```python
from build123d import *

# Parameters (mm, degrees)
SKETCH1_W                       = 361.95
SKETCH1_H                       = 110.744
BOSS_EXTRUDE1_DEPTH             = 3.175
CUT_EXTRUDE1_DEPTH              = 379.526243028
SKETCH3_W                       = 36.5125
SKETCH3_H                       = 28.575
CUT_EXTRUDE2_DEPTH              = 379.526243028
FILLET1_R                       = 6.35
F_1_4_CLEARANCE_HOLE1_OUTLINE_R = 3.3782
F_1_4_CLEARANCE_HOLE1_DEPTH     = 3.175
CUT_EXTRUDE6_DEPTH              = 3.175


# Read off the part's stored shape, not the designer's step: 1/4 Clearance Hole1, Cut-Extrude6
with BuildPart() as part:
    # Sketch1 → Boss-Extrude1 (new body)
    with BuildSketch(Plane(origin=(0, 0, 0), x_dir=(1, 0, 0), z_dir=(0, 1, 0))):
        with Locations((180.975, 55.372)):
            Rectangle(SKETCH1_W, SKETCH1_H)
    extrude(amount=BOSS_EXTRUDE1_DEPTH)

    # Sketch2 → Cut-Extrude1 (cut, through all)
    with BuildSketch(Plane(origin=(0, 3.175, 0), x_dir=(1, 0, 0), z_dir=(0, 1, 0))):
        Polygon((0, 0), (31.233038214, 110.744), (0, 110.744), align=None)
        Polygon((361.95, 0), (307.33710294, 110.744), (361.95, 110.744), align=None)
    extrude(amount=-CUT_EXTRUDE1_DEPTH, mode=Mode.SUBTRACT)

    # Sketch3 → Cut-Extrude2 (cut, through all)
    with BuildSketch(Plane(origin=(0, 3.175, 0), x_dir=(1, 0, 0), z_dir=(0, 1, 0))):
        with Locations((57.15, 96.4565)):
            Rectangle(SKETCH3_W, SKETCH3_H)
        with Locations((285.75, 96.4565)):
            Rectangle(SKETCH3_W, SKETCH3_H)
    extrude(amount=-CUT_EXTRUDE2_DEPTH, mode=Mode.SUBTRACT)

    # Fillet1
    fillet1_edges = [part.edges().sort_by_distance(p)[0] for p in [
        (75.40625, 1.5875, -82.169),
        (38.89375, 1.5875, -82.169),
        (304.00625, 1.5875, -82.169),
        (267.49375, 1.5875, -82.169),
    ]]
    fillet(fillet1_edges, radius=FILLET1_R)

    # 1/4 Clearance Hole1 outline → 1/4 Clearance Hole1 (cut)
    with BuildSketch(Plane(origin=(0, 0, 0), x_dir=(1, 0, 0), z_dir=(0, 1, 0))):
        with BuildLine():
            ThreePointArc((51.7525, 23.01875), (56.1975, 18.57375), (60.6425, 23.01875))
            Line((60.6425, 23.01875), (60.6425, 27.78125))
            ThreePointArc((60.6425, 27.78125), (56.1975, 32.22625), (51.7525, 27.78125))
            Line((51.7525, 27.78125), (51.7525, 23.01875))
        make_face()
        with Locations((297.65625, 23.314421689)):
            Circle(F_1_4_CLEARANCE_HOLE1_OUTLINE_R)
        with Locations((297.65625, 42.364421689)):
            Circle(F_1_4_CLEARANCE_HOLE1_OUTLINE_R)
        with Locations((45.24375, 23.314421689)):
            Circle(F_1_4_CLEARANCE_HOLE1_OUTLINE_R)
        with Locations((45.24375, 42.364421689)):
            Circle(F_1_4_CLEARANCE_HOLE1_OUTLINE_R)
    extrude(amount=F_1_4_CLEARANCE_HOLE1_DEPTH, mode=Mode.SUBTRACT)

    # Cut-Extrude6 outline → Cut-Extrude6 (cut)
    with BuildSketch(Plane(origin=(0, 0, 0), x_dir=(1, 0, 0), z_dir=(0, 1, 0))):
        with BuildLine():
            ThreePointArc((39.02075, 71.1835), (39.8145, 71.97725), (39.02075, 72.771))
            Line((39.02075, 72.771), (32.41675, 72.771))
            ThreePointArc((32.41675, 72.771), (31.623, 71.97725), (32.41675, 71.1835))
            Line((32.41675, 71.1835), (32.41675, 39.240862815))
            ThreePointArc((32.41675, 39.240862815), (31.623, 38.447112815), (32.41675, 37.653362815))
            Line((32.41675, 37.653362815), (39.02075, 37.653362815))
            ThreePointArc((39.02075, 37.653362815), (39.8145, 38.447112815), (39.02075, 39.240862815))
            Line((39.02075, 39.240862815), (39.02075, 71.1835))
        make_face()
        with BuildLine():
            ThreePointArc((310.48325, 71.1835), (311.277, 71.97725), (310.48325, 72.771))
            Line((310.48325, 72.771), (303.87925, 72.771))
            ThreePointArc((303.87925, 72.771), (303.0855, 71.97725), (303.87925, 71.1835))
            Line((303.87925, 71.1835), (303.87925, 39.240862815))
            ThreePointArc((303.87925, 39.240862815), (303.0855, 38.447112815), (303.87925, 37.653362815))
            Line((303.87925, 37.653362815), (310.48325, 37.653362815))
            ThreePointArc((310.48325, 37.653362815), (311.277, 38.447112815), (310.48325, 39.240862815))
            Line((310.48325, 39.240862815), (310.48325, 71.1835))
        make_face()
    extrude(amount=CUT_EXTRUDE6_DEPTH, mode=Mode.SUBTRACT)


solid = part.part
```
Work out the finished part from the listing and answer in its coordinate system (mm). A direction names the side the tool comes from. Give positions to 0.01 mm unless a question says otherwise; leave off trailing zeros. Order: outer loops, then holes, each group sorted by start corner. A loop starts at its lowest first (then second) coordinate and runs counter-clockwise, first axis right, second up. Notation, with made-up numbers: M 74,-5 L 118,-5 A19 ccw 118,2 Z; hole C 55.5,30.25 d1. An arc over 180 degrees is marked long. Return JSON: item names as keys, results as strings.
1) Each of these flat-tipped pins is pushed along its axis until it touches: pin 1 (1.6 mm diameter, centred on y = 1, z = -26, fed in from +X); pin 2 (1 mm diameter, centred on x = 289, y = 1, fed in from -Z); pin 3 (1 mm diameter, centred on x = 46, z = -41.5, fed in from +Y); pin 4 (1 mm diameter, centred on y = 2, z = -53.5, fed in from +X). Where does it stop, or does it pass through?
Resolved:
{"pin 1": "x = 349.52", "pin 2": "z = -82.17", "pin 3": "through", "pin 4": "x = 335.81"}
2) Section C-C, the plane y = 1.85 is taken. Give the number of separate pieces and of enclosed holes in the cut face, plus the area to 3 significant figures.
Resolved:
{"separate pieces": "1", "enclosed holes": "7", "area": "32,600 mm^2"}
3) Section B-B, the plane z = -61 is taken. Write down the section's boundary in (x, y) (3 decimals).
Resolved:
{"outline": "M 17.204,0 L 32.417,0 L 32.417,3.175 L 17.204,3.175 Z; M 39.021,0 L 303.879,0 L 303.879,3.175 L 39.021,3.175 Z; M 310.483,0 L 331.868,0 L 331.868,3.175 L 310.483,3.175 Z"}
4) A tool of negligible diameter and unlimited length cuts with its end or side. For faces 1 (the flat face through (15.4, 1.6, -54.6)), 2 (the cylindrical face through (73.497, 1.565, -83.98)), from which of +Z, -Z, +X, -X, +Y, -Y can it reach the whole face along a straight path? Write none if from no direction.
Resolved:
{"face 1": "-Z, -X, +Y, -Y", "face 2": "-Z, +Y, -Y"}
5) Straight lines are drawn through the part: line 1 along Z through (x, y) = (298, 2.25); line 2 along X through (y, z) = (0.3, -57); line 3 along X through (y, z) = (1.05, -83). For each, find the intervals that lie inside material, in ascending order. Write a range as [from, to].
Resolved:
{"line 1": "[-82.18, -45.73], [-39, -26.68], [-19.95, 0]", "line 2": "[16.08, 32.42], [39.02, 303.88], [310.48, 333.84]", "line 3": "[23.41, 42.1], [72.2, 270.7], [300.8, 321.02]"}
6) For a pull along X with two mould halves and no side action, classify faces 3 (the flat face through (335.026, 1.61, -54.597)), 4 (the flat face through (178, 0, -56)), 5 (the cylindrical face through (294.28, 1.57, -23.46)) as +X half, -X half, draft (parallel to the pull), parting line (faces both ways), or undercut.
Resolved:
{"face 3": "+X half", "face 4": "draft", "face 5": "undercut"}
7) Section D-D, the plane z = -10 is taken. Write down the section's boundary in (x, y) (3 decimals).
Resolved:
{"outline": "M 2.82,0 L 357.019,0 L 357.019,3.175 L 2.82,3.175 Z"}
8) Section A-A, the plane z = -94 is taken. Write down the section's boundary in (x, y) (3 decimals).
Resolved:
{"outline": "M 26.511,0 L 38.894,0 L 38.894,3.175 L 26.511,3.175 Z; M 75.406,0 L 267.494,0 L 267.494,3.175 L 75.406,3.175 Z; M 304.006,0 L 315.594,0 L 315.594,3.175 L 304.006,3.175 Z"}
